The figure shows three views and two pictorial views of one solid part (mm, origin at its lowest corner). Answer the questions. A direction names the side the tool comes from. Round coordinates to 2 decimals unless told otherwise and drop trailing zeros. Order: outer loops, then holes, each group sorted by start corner. A loop starts at its lowest first (then second) coordinate and runs counter-clockwise, first axis right, second up. Notation, with made-up numbers: (-13, 84) - (12, 84) arc R29 ccw to (12, 106) - close; hole circle Ø1 at (65.25, 23.25). An arc over 180 degrees is marked (long way). Answer as a JSON object with one key per item and string values. Group by question number.
Q1. A cutting plane is placed at A-A on z = 14. Determine the outline of the cut face in (x, y).
Q2. Given pin 1 Ø1.5 at (x, y) = (1.5, 10) entering from -Z; pin 2 Ø11 at (y, z) = (11.5, 17) entering from +X; pin 3 Ø1 at (y, z) = (22.5, 21.5) entering from +X; pin 4 Ø2 at (x, y) = (2, 25) entering from +Z, each flat-ended and moving along its own axis, determine where each tip first touches the part or whether it passes through.
Q3. A cutting plane is placed at B-B on y = 14.75. Determine the outline of the cut face in (x, z) (1 decimal).
Q4. The mould has two halves that part along Z. Classify the marked faces 1, 2 and 3: pulls with the +Z half, pulls with the -Z half, needs draft (parallel to the pull), parting line crosses it, or undercut.
Q5. A cutting plane is placed at D-D on z = 21. Determine the outline of the cut face in (x, y).
Q6. A tool of negligible diameter and unlimited length cuts with its end or side. For the marked faces 4, 5 and 6, from which of +Z, -Z, +X, -X, +Y, -Y can it reach the whole face along a straight path? Write none if from no direction.
Q7. A cutting plane is placed at C-C on x = 0.35. Count the separate pieces of the cut face and the enclosed holes in it, and give its area (3 significant figures).
Q8. Consider line 1 (Y direction, x = 2.65, z = 14); line 2 (Z direction, x = 1.9, y = 15.75) (1 decimal); line 3 (Z direction, x = 0.4, y = 4.5) (1 decimal). Determine where each line is inside the solid, lowest interval first.
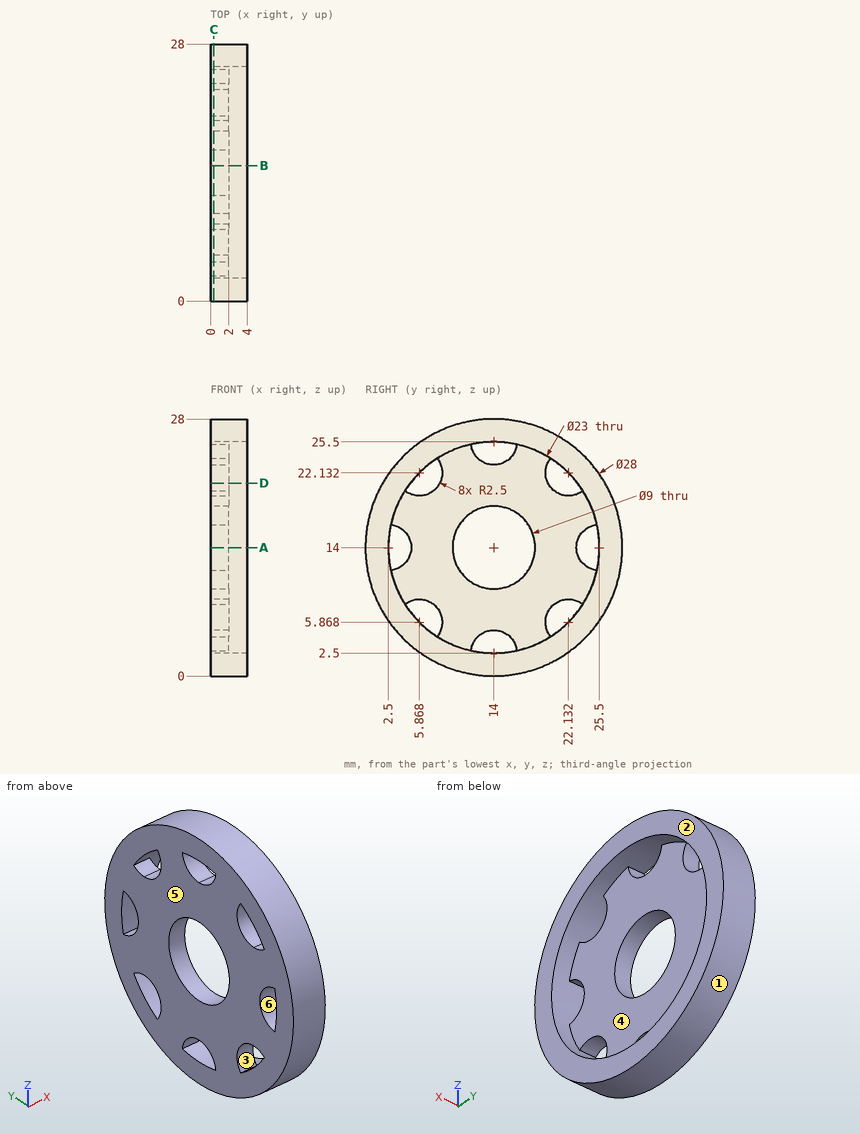
Result set:
{
 "1": {"outline": "(0, 0) - (4, 0) - (4, 2.5) - (0, 2.5) - close; (0, 5) - (2, 5) - (2, 9.5) - (0, 9.5) - close; (0, 18.5) - (2, 18.5) - (2, 23) - (0, 23) - close; (0, 25.5) - (4, 25.5) - (4, 28) - (0, 28) - close"},
 "2": {"pin 1": "stops at z = 0.38", "pin 2": "stops at x = 2", "pin 3": "stops at x = 4", "pin 4": "stops at z = 23.8"},
 "3": {"outline": "(0, 0) - (4, 0) - (4, 2.5) - (0, 2.5) - close; (0, 4.9) - (2, 4.9) - (2, 9.6) - (0, 9.6) - close; (0, 18.4) - (2, 18.4) - (2, 23.1) - (0, 23.1) - close; (0, 25.5) - (4, 25.5) - (4, 28) - (0, 28) - close"},
 "4": {"face 1": "parting line crosses it", "face 2": "needs draft", "face 3": "undercut"},
 "5": {"outline": "(0, 1.88) - (4, 1.88) - (4, 4.88) - (0, 4.88) - close; (0, 8.1) - (2, 8.1) - (2, 19.9) - (0, 19.9) - close; (0, 23.12) - (4, 23.12) - (4, 26.12) - (0, 26.12) - close"},
 "6": {"face 4": "+X", "face 5": "+Z, -Z, -X, +Y, -Y", "face 6": "+X, -X"},
 "7": {"separate pieces": "1", "enclosed holes": "9", "area": "477 mm²"},
 "8": {"line 1": "y = 0 to 2.5, 25.5 to 28", "line 2": "z = 0.1 to 2.6, 4.3 to 9.9, 18.1 to 23.7, 25.4 to 27.9", "line 3": "z = 3.7 to 7.5, 8 to 12.5, 15.5 to 20, 20.5 to 24.3"}
}
